```python
from build123d import *

# Parameters (mm, degrees)
BOSS_EXTRUDE1_DEPTH = 3
CUT_EXTRUDE1_REACH  = 77.661
SKETCH1_3_R         = 1.25
BOSS_EXTRUDE2_START = 8.86
BOSS_EXTRUDE2_DEPTH = 8.86
BOSS_EXTRUDE3_START = 1.5
SKETCH1_5_R         = 3.21
SKETCH1_5_R_2       = 1.25
BOSS_EXTRUDE3_DEPTH = 1.5
SKETCH2_W           = 12.28
SKETCH2_H           = 8.73
CUT_EXTRUDE2_DEPTH  = 3
BOSS_EXTRUDE7_DEPTH = 5
FILLET4_R           = 1


with BuildPart() as part:
    # Sketch1 → Boss-Extrude1 (new body)
    with BuildSketch(Plane(origin=(0, 0, 0), x_dir=(1, 0, 0), z_dir=(0, 1, 0))):
        with BuildLine():
            Line((3.81, 3), (49.09, 3))
            ThreePointArc((49.09, 3), (53.90539718, 1.00539718), (55.9, -3.81))
            Line((55.9, -3.81), (55.9, -44.09))
            ThreePointArc((55.9, -44.09), (53.90539718, -48.90539718), (49.09, -50.9))
            Line((49.09, -50.9), (3.81, -50.9))
            ThreePointArc((3.81, -50.9), (-1.00539718, -48.90539718), (-3, -44.09))
            Line((-3, -44.09), (-3, -3.81))
            ThreePointArc((-3, -3.81), (-1.00539718, 1.00539718), (3.81, 3))
        make_face()
    extrude(amount=-BOSS_EXTRUDE1_DEPTH)

    # Sketch1_3 → Cut-Extrude1 (cut, up to next)
    with BuildSketch(Plane(origin=(0, 0, 0), x_dir=(1, 0, 0), z_dir=(0, 1, 0)), mode=Mode.PRIVATE) as cut_extrude1_sk1:
        with Locations(Location((3.81, -3.81, 0), (0, 0, 270))):
            Circle(SKETCH1_3_R)
    cut_extrude1_tool1 = extrude(cut_extrude1_sk1.sketch, amount=-CUT_EXTRUDE1_REACH, mode=Mode.PRIVATE) & part.part
    # Sketch1_3 → Cut-Extrude1 (cut, up to next)
    with BuildSketch(Plane(origin=(0, 0, 0), x_dir=(1, 0, 0), z_dir=(0, 1, 0)), mode=Mode.PRIVATE) as cut_extrude1_sk2:
        with Locations(Location((3.81, -44.09, 0), (0, 0, 270))):
            Circle(SKETCH1_3_R)
    cut_extrude1_tool2 = extrude(cut_extrude1_sk2.sketch, amount=-CUT_EXTRUDE1_REACH, mode=Mode.PRIVATE) & part.part
    # Sketch1_3 → Cut-Extrude1 (cut, up to next)
    with BuildSketch(Plane(origin=(0, 0, 0), x_dir=(1, 0, 0), z_dir=(0, 1, 0)), mode=Mode.PRIVATE) as cut_extrude1_sk3:
        with Locations(Location((49.09, -44.09, 0), (0, 0, 270))):
            Circle(SKETCH1_3_R)
    cut_extrude1_tool3 = extrude(cut_extrude1_sk3.sketch, amount=-CUT_EXTRUDE1_REACH, mode=Mode.PRIVATE) & part.part
    # Sketch1_3 → Cut-Extrude1 (cut, up to next)
    with BuildSketch(Plane(origin=(0, 0, 0), x_dir=(1, 0, 0), z_dir=(0, 1, 0)), mode=Mode.PRIVATE) as cut_extrude1_sk4:
        with Locations(Location((49.09, -3.81, 0), (0, 0, 270))):
            Circle(SKETCH1_3_R)
    cut_extrude1_tool4 = extrude(cut_extrude1_sk4.sketch, amount=-CUT_EXTRUDE1_REACH, mode=Mode.PRIVATE) & part.part
    add(cut_extrude1_tool1.solids().sort_by_distance((3.81, 0, 3.81))[0], mode=Mode.SUBTRACT)
    add(cut_extrude1_tool2.solids().sort_by_distance((3.81, 0, 44.09))[0], mode=Mode.SUBTRACT)
    add(cut_extrude1_tool3.solids().sort_by_distance((49.09, 0, 44.09))[0], mode=Mode.SUBTRACT)
    add(cut_extrude1_tool4.solids().sort_by_distance((49.09, 0, 3.81))[0], mode=Mode.SUBTRACT)

    # Sketch1_4 → Boss-Extrude2 (add)
    with BuildSketch(Plane(origin=(0, 0, 0), x_dir=(1, 0, 0), z_dir=(0, 1, 0)).offset(BOSS_EXTRUDE2_START)):
        with BuildLine():
            ThreePointArc((-3, -3.81), (-1.00539718, 1.00539718), (3.81, 3))
            Line((3.81, 3), (49.09, 3))
            ThreePointArc((49.09, 3), (53.90539718, 1.00539718), (55.9, -3.81))
            Line((55.9, -3.81), (55.9, -44.09))
            ThreePointArc((55.9, -44.09), (53.90539718, -48.90539718), (49.09, -50.9))
            Line((49.09, -50.9), (3.81, -50.9))
            ThreePointArc((3.81, -50.9), (-1.00539718, -48.90539718), (-3, -44.09))
            Line((-3, -44.09), (-3, -3.81))
        make_face()
        with BuildLine():
            Line((52.9, -3.81), (52.9, -44.09))
            ThreePointArc((52.9, -44.09), (51.784076836, -46.784076836), (49.09, -47.9))
            Line((49.09, -47.9), (3.81, -47.9))
            ThreePointArc((3.81, -47.9), (1.115923164, -46.784076836), (0, -44.09))
            Line((0, -44.09), (0, -3.81))
            ThreePointArc((0, -3.81), (1.115923164, -1.115923164), (3.81, 0))
            Line((3.81, 0), (49.09, 0))
            ThreePointArc((49.09, 0), (51.784076836, -1.115923164), (52.9, -3.81))
        make_face(mode=Mode.SUBTRACT)
    extrude(amount=-BOSS_EXTRUDE2_DEPTH)

    # Sketch1_5 → Boss-Extrude3 (add)
    # profile 1 of 4: a face of its own
    with BuildSketch(Plane(origin=(0, 0, 0), x_dir=(1, 0, 0), z_dir=(0, 1, 0)).offset(BOSS_EXTRUDE3_START)):
        with Locations(Location((49.09, -3.81, 0), (0, 0, 90))):
            Circle(SKETCH1_5_R)
        with Locations(Location((49.09, -3.81, 0), (0, 0, 270))):
            Circle(SKETCH1_5_R_2, mode=Mode.SUBTRACT)
    # profile 2 of 4: a face of its own
    with BuildSketch(Plane(origin=(0, 0, 0), x_dir=(1, 0, 0), z_dir=(0, 1, 0)).offset(BOSS_EXTRUDE3_START)):
        with Locations(Location((49.09, -44.09, 0), (0, 0, 90))):
            Circle(SKETCH1_5_R)
        with Locations(Location((49.09, -44.09, 0), (0, 0, 270))):
            Circle(SKETCH1_5_R_2, mode=Mode.SUBTRACT)
    # profile 3 of 4: a face of its own
    with BuildSketch(Plane(origin=(0, 0, 0), x_dir=(1, 0, 0), z_dir=(0, 1, 0)).offset(BOSS_EXTRUDE3_START)):
        with Locations(Location((3.81, -44.09, 0), (0, 0, 90))):
            Circle(SKETCH1_5_R)
        with Locations(Location((3.81, -44.09, 0), (0, 0, 270))):
            Circle(SKETCH1_5_R_2, mode=Mode.SUBTRACT)
    # profile 4 of 4: a face of its own
    with BuildSketch(Plane(origin=(0, 0, 0), x_dir=(1, 0, 0), z_dir=(0, 1, 0)).offset(BOSS_EXTRUDE3_START)):
        with Locations(Location((3.81, -3.81, 0), (0, 0, 90))):
            Circle(SKETCH1_5_R)
        with Locations(Location((3.81, -3.81, 0), (0, 0, 270))):
            Circle(SKETCH1_5_R_2, mode=Mode.SUBTRACT)
    extrude(amount=-BOSS_EXTRUDE3_DEPTH)

    # Sketch2 → Cut-Extrude2 (cut)
    with BuildSketch(Plane.XY.offset(50.9)):
        with Locations((18.5, 4.5)):
            Rectangle(SKETCH2_W, SKETCH2_H)
    extrude(amount=-CUT_EXTRUDE2_DEPTH, mode=Mode.SUBTRACT)

    # Sketch8 → Boss-Extrude7 (add)
    with BuildSketch(Plane.XZ.offset(3)):
        with BuildLine():
            Line((47.9, 50.9), (30.15, 50.9))
            Line((30.15, 50.9), (30.15, 59.78))
            ThreePointArc((30.15, 59.78), (31.292283553, 62.537716447), (34.05, 63.68))
            Line((34.05, 63.68), (44, 63.68))
            ThreePointArc((44, 63.68), (46.757716447, 62.537716447), (47.9, 59.78))
            Line((47.9, 59.78), (47.9, 50.9))
        make_face()
        with BuildLine():
            Line((41.9, 53.9), (36.15, 53.9))
            ThreePointArc((36.15, 53.9), (34.028679656, 54.778679656), (33.15, 56.9))
            Line((33.15, 56.9), (33.15, 57.68))
            ThreePointArc((33.15, 57.68), (34.028679656, 59.801320344), (36.15, 60.68))
            Line((36.15, 60.68), (41.9, 60.68))
            ThreePointArc((41.9, 60.68), (44.021320344, 59.801320344), (44.9, 57.68))
            Line((44.9, 57.68), (44.9, 56.9))
            ThreePointArc((44.9, 56.9), (44.021320344, 54.778679656), (41.9, 53.9))
        make_face(mode=Mode.SUBTRACT)
    extrude(amount=-BOSS_EXTRUDE7_DEPTH)

    # Fillet4
    fillet4_edges = [part.edges().sort_by_distance(p)[0] for p in [
        (47.9, 2, 55.34),
        (30.15, 2, 55.34),
        (31.292283553, 2, 62.537716447),
        (39.025, 2, 63.68),
        (46.757716447, 2, 62.537716447),
        (39.025, 2, 60.68),
        (34.028679656, 2, 59.801320344),
        (33.15, 2, 57.29),
        (34.028679656, 2, 54.778679656),
        (39.025, 2, 53.9),
        (44.021320344, 2, 54.778679656),
        (44.9, 2, 57.29),
        (44.021320344, 2, 59.801320344),
    ]]
    fillet(fillet4_edges, radius=FILLET4_R)


solid = part.part
```
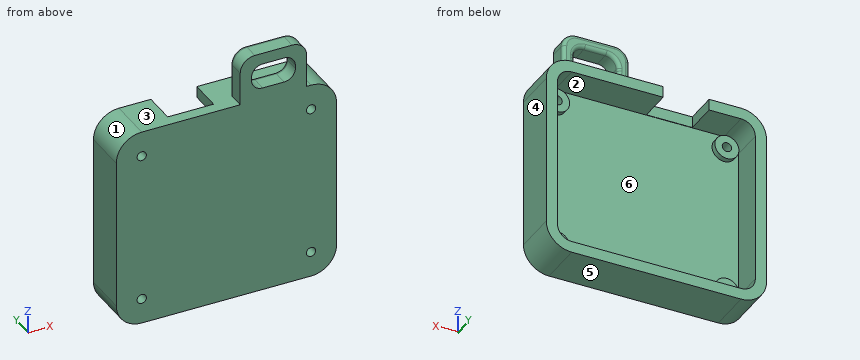
Source: CAD feature listing. Evaluate the final solid. Frame: model axes, mm. Face numbers are marked on the shaded views. A direction names the side the tool comes from. Coordinates: 2 decimals unless noted, no trailing zeros. Write each loop counter-clockwise with the first axis right and the second up, starting at its lowest first coordinate (ties: lowest second). Pieces come first, ordered by that corner, then holes. Notation, with made-up numbers: M 75.5,74.5 L 93.5,74.5 A24 ccw 93.5,97.5 Z; hole C 79.25,9.25 d5. An arc over 180 degrees is marked long. Answer as a JSON object with one key per item and string values.
1. Cut plane B-B on y = 5. Output: boundary loops of the cut face in (x, z), plus the area to 3 significant figures.
Evaluation:
{"outline": "M -3,3.81 A6.81 ccw 3.81,-3 L 49.09,-3 A6.81 ccw 55.9,3.81 L 55.9,44.09 A6.81 ccw 49.09,50.9 L 24.64,50.9 L 24.64,47.9 L 49.09,47.9 A3.81 cw 52.9,44.09 L 52.9,3.81 A3.81 cw 49.09,0 L 3.81,0 A3.81 cw 0,3.81 L 0,44.09 A3.81 cw 3.81,47.9 L 12.36,47.9 L 12.36,50.9 L 3.81,50.9 A6.81 ccw -3,44.09 Z", "area": "577 mm^2"}
2. Ray query, L1, parallel to X at y = -1.7, z = 3.81; L2, parallel to X at y = 0.2, z = 3.81; L3, parallel to X at y = 6.5, z = 19. Return the intervals inside material, ascending.
Evaluation:
{"L1": "-3 to 2.56, 5.06 to 47.84, 50.34 to 55.9", "L2": "-3 to 0, 0.6 to 2.56, 5.06 to 7.02, 45.88 to 47.84, 50.34 to 52.3, 52.9 to 55.9", "L3": "-3 to 0, 52.9 to 55.9"}
3. Cut plane C-C on z = 33. Output: boundary loops of the cut face in (x, y).
Evaluation:
{"outline": "M -3,-3 L 55.9,-3 L 55.9,8.86 L 52.9,8.86 L 52.9,0 L 0,0 L 0,8.86 L -3,8.86 Z"}
4. Contact query for flat-ended pins moving along their axis: P1, Ø1.5, axis at y = 0, z = 47.5, coming from the -X side; P2, Ø6, axis at y = 0.5, z = 55, coming from the -X side; P3, Ø3, axis at y = -0.5, z = 56.5, coming from the +X side; P4, Ø3, axis at x = 49.09, z = 3.81, coming from the -Y side. Output: stop coordinate, or through.
Evaluation:
{"P1": "x = -2.46", "P2": "x = 30.15", "P3": "x = 47.9", "P4": "y = -3"}
5. Cut plane A-A on x = 14.5. Output: boundary loops of the cut face in (y, z) (3 decimals), plus the area to 3 significant figures.
Evaluation:
{"outline": "M -3,-3 L 8.86,-3 L 8.86,0 L 0,0 L 0,47.9 L 0.135,47.9 L 0.135,50.9 L -3,50.9 Z", "area": "189 mm^2"}
6. Draft query along X for the marked faces 1, 2, 3 and 4. Return one class per face: released by +X, released by -X, zero draft, split by the parting line, or undercut.
Evaluation:
{"face 1": "released by -X", "face 2": "undercut", "face 3": "zero draft", "face 4": "released by +X"}
7. Access query for the marked faces 5 and 6. Directions: +Z, -Z, +X, -X, +Y, -Y. A direction counts if a zero-diameter tool reaches every point of the face in a straight line with its end or side. Return the directions, or none.
Evaluation:
{"face 5": "-Z, +X, -X, +Y, -Y", "face 6": "+Y"}
